Part model, mm, in its own coordinate system. Face numbers are marked on the shaded views. A direction names the side the tool comes from. Give positions to 0.01 mm unless a question says otherwise; leave off trailing zeros. Write each loop counter-clockwise with the first axis right and the second up, starting at its lowest first coordinate (ties: lowest second). Pieces come first, ordered by that corner, then holes. Notation, with made-up numbers: M -1,-23 L 54,-23 A13 cw 54,-2 Z; hole C 47,14.25 d2. An arc over 180 degrees is marked long. Use CSV: the item, a comma, the result in double quotes. Start each with the question number.
1. Mould opens along X. For the marked faces 1, 2 and 3 say: pulls with the +X half, pulls with the -X half, needs draft (parallel to the pull), parting line crosses it, or undercut.
2. Drop flat-ended pins along their axis: pin 1 Ø5 at (x, z) = (32.5, -10.5) entering from +Y; pin 2 Ø6 at (x, z) = (41, -8) entering from -Y; pin 3 Ø2 at (x, y) = (41.5, 50) entering from +Z. Give the stop position or say it passes through.
3. Band-saw the part on D-D, the plane z = -18. Count the separate pieces of the cut face and the enclosed holes in it, then the cut area to 3 significant figures.
4. Band-saw the part on B-B, the plane y = 24. List the corners of the cut face in (x, z).
5. 3-axis set-ups, long thin cutter, end or side, ignore diameter. For the marked faces 4, 5, 6 and 7: which of +Z, -Z, +X, -X, +Y, -Y reach the whole face in a straight line?
6. Drill centre lines: line 1 along Y through (x, z) = (36.5, -2.5); line 2 along Y through (x, z) = (5, -18); line 3 along Z through (x, y) = (35, 42). Where is each one in solid material? Low to high. Write a range as from..to.
7. Band-saw the part on A-A, the plane y = 12.5. List the corners of the cut face in (x, z), then the cut area to 3 significant figures.
8. Band-saw the part on C-C, the plane y = 32. List the corners of the cut face in (x, z).
from build123d import *

# Parameters (mm, degrees)
SCHIZZO1_R                   = 2
SCHIZZO1_R_2                 = 1.55
SCHIZZO1_R_3                 = 6.25
ESTRUSIONE_ESTRUSIONE1_DEPTH = 20
TAGLIO_ESTRUSIONE3_DEPTH     = 16
SCHIZZO5_R                   = 1.75
TAGLIO_ESTRUSIONE4_DEPTH     = 68.079836494


with BuildPart() as part:
    # Schizzo1 → Estrusione-Estrusione1 (new body)
    with BuildSketch(Plane.XY):
        with BuildLine():
            Line((0, 0), (30.205221293, 0))
            Line((30.205221293, 0), (30.205221293, 25.000000003))
            Line((30.205221293, 25.000000003), (50, 25.000000003))
            Line((50, 25.000000003), (50, 46.083449556))
            add(Edge.make_bspline(
                [(10, 45.902878326), (10, 53.523029111), (16.665197751, 64.749431614), (39.917897707, 66.566627657), (50, 55.41391796), (50, 46.083449556)],
                knots=[0, 0, 0, 0, 0.305409074, 0.638645938, 1, 1, 1, 1], degree=3))
            Line((10, 45.902878326), (10, 25))
            Line((10, 25), (0, 25))
            Line((0, 25), (0, 0))
        make_face()
        with Locations((5.830221293, 7.000447051)):
            Circle(SCHIZZO1_R, mode=Mode.SUBTRACT)
        with Locations((13.955221293, 12.5)):
            Circle(SCHIZZO1_R, mode=Mode.SUBTRACT)
        with Locations((22.080221293, 7.000447051)):
            Circle(SCHIZZO1_R, mode=Mode.SUBTRACT)
        with Locations((22.080221293, 19.500447051)):
            Circle(SCHIZZO1_R, mode=Mode.SUBTRACT)
        with Locations((5.830221293, 19.500447051)):
            Circle(SCHIZZO1_R, mode=Mode.SUBTRACT)
        with Locations((37.899494937, 55.899494937)):
            Circle(SCHIZZO1_R_2, mode=Mode.SUBTRACT)
        with Locations((28, 46)):
            Circle(SCHIZZO1_R_3, mode=Mode.SUBTRACT)
        with Locations((18.100505063, 36.100505063)):
            Circle(SCHIZZO1_R_2, mode=Mode.SUBTRACT)
        with Locations((18.100505063, 55.899494937)):
            Circle(SCHIZZO1_R_2, mode=Mode.SUBTRACT)
    extrude(amount=-ESTRUSIONE_ESTRUSIONE1_DEPTH)

    # Schizzo4 → Taglio-Estrusione3 (cut)
    with BuildSketch(Plane.XY):
        Polygon((42.707691964, 34.412315024), (50, 34.412315024), (50, 57.587684976), (50, 63.39531064), (42.707691964, 63.39531064), (42.707691964, 57.587684976), (33.442882673, 48.113516989), (33.442882673, 43.886483011), align=None)
    extrude(amount=-TAGLIO_ESTRUSIONE3_DEPTH, mode=Mode.SUBTRACT)

    # Schizzo5 → Taglio-Estrusione4 (cut, through all)
    with BuildSketch(Plane(origin=(0, 25.000000003, 0), x_dir=(1, 0, 0), z_dir=(0, 1, 0))):
        with Locations(Location((34.937925583, 8, 0), (0, 0, 90))):
            Circle(SCHIZZO5_R)
    extrude(amount=TAGLIO_ESTRUSIONE4_DEPTH, mode=Mode.SUBTRACT)


solid = part.part
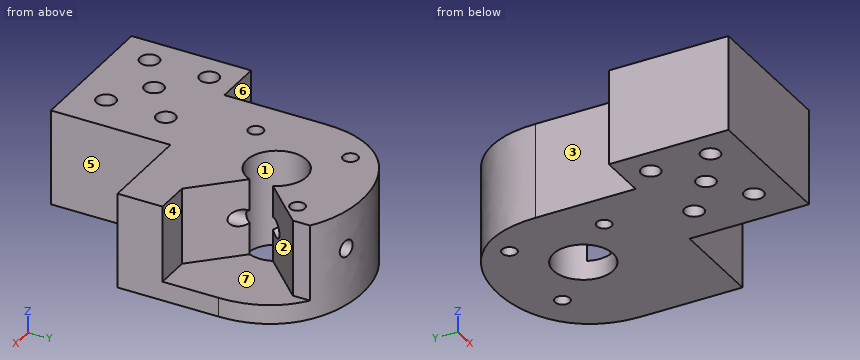
Output:
1,face 1,"undercut"
1,face 2,"pulls with the +X half"
1,face 3,"pulls with the -X half"
2,pin 1,"stops at y = 65"
2,pin 2,"stops at y = 25"
2,pin 3,"stops at z = -16"
3,separate pieces,"1"
3,enclosed holes,"9"
3,area,"2,000 mm²"
4,outline,"M 0,-20 L 30.21,-20 L 30.21,0 L 0,0 Z"
5,face 4,"+Z, +X, +Y"
5,face 5,"+Z, -Z, +X, -Y"
5,face 6,"+Z, -Z, -X, +Y"
5,face 7,"+Z, +X"
6,line 1,"y = 25..40.76, 51.24..55.23, 56.57..64.09"
6,line 2,"y = 0..5.18, 8.82..17.68, 21.32..25"
6,line 3,"z = -20..-9.75, -6.25..0"
7,outline,"M 0,-20 L 11.96,-20 L 11.96,0 L 0,0 Z; M 15.96,-20 L 30.21,-20 L 30.21,0 L 15.96,0 Z"
7,area,"524 mm²"
8,outline,"M 10,-20 L 50,-20 L 50,0 L 10,0 Z; hole C 34.94,-8 d3.5"
